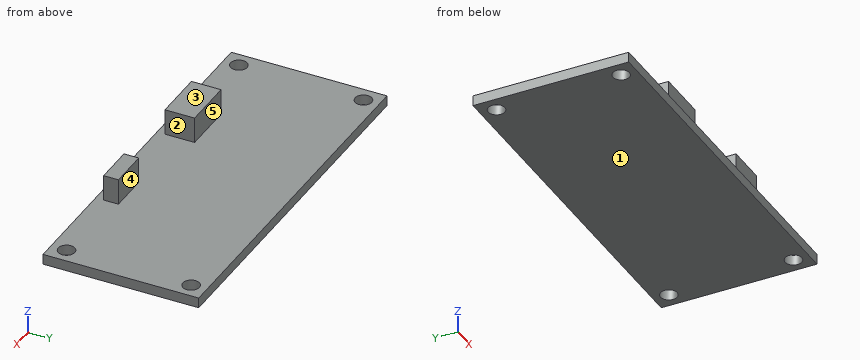
```python
from build123d import *

# Parameters (mm, degrees)
SKETCH_1_W      = 71
SKETCH_1_H      = 30
SKETCH_1_R      = 1.6
EXTRUDE_1_DEPTH = 2
SKETCH_2_W      = 9.975674075
SKETCH_2_H      = 5.707731043
SKETCH_2_W_2    = 7.661729058
SKETCH_2_H_2    = 2.853865522
EXTRUDE_2_DEPTH = 5


with BuildPart() as part:
    # 草图1 → 凸台-拉伸1 (new body)
    with BuildSketch(Plane.XY):
        with Locations((35.5, 15)):
            Rectangle(SKETCH_1_W, SKETCH_1_H)
        with Locations((3, 27)):
            Circle(SKETCH_1_R, mode=Mode.SUBTRACT)
        with Locations((68, 3)):
            Circle(SKETCH_1_R, mode=Mode.SUBTRACT)
        with Locations((3, 3)):
            Circle(SKETCH_1_R, mode=Mode.SUBTRACT)
        with Locations((68, 27)):
            Circle(SKETCH_1_R, mode=Mode.SUBTRACT)
    extrude(amount=EXTRUDE_1_DEPTH)

    # 草图2 → 凸台-拉伸2 (add)
    with BuildSketch(Plane.XY.offset(2)):
        with Locations((23.004696906, 4.381563419)):
            Rectangle(SKETCH_2_W, SKETCH_2_H)
        with Locations((47.301119589, 2.954630659)):
            Rectangle(SKETCH_2_W_2, SKETCH_2_H_2)
    extrude(amount=EXTRUDE_2_DEPTH)


solid = part.part
```
CAD build for the part. Positions are in the model's coordinates, mm. Face numbers are marked on the shaded views. A direction names the side the tool comes from. Coordinates: 2 decimals unless noted, no trailing zeros. Order: outer loops, then holes, each group sorted by start corner. A loop starts at its lowest first (then second) coordinate and runs counter-clockwise, first axis right, second up. Notation, with made-up numbers: M 27.25,-8 L 83.25,-8 A11 cw 83.25,0 Z; hole C 1,57 d9. An arc over 180 degrees is marked long. Write each question's results on one line, items separated by ' | '. Start each with the question number.
Q1. Cut at B-B (y = 27). List the corners of the cut face in (x, z), then the cut area to 3 significant figures.
Q2. Cut at C-C (z = 3). List the corners of the cut face in (x, y), then the cut area to 3 significant figures.
Q3. Cut at A-A (x = 68). List the corners of the cut face in (y, z).
Q4. Which spindle directions (+Z, -Z, +X, -X, +Y, -Y) get a long thin tool onto all of the face, cutting with end or side? Do the marked faces 3, 4 and 5. Say none if no direction does.
Q5. Drill centre lines: probe 1 along Y at (x, z) = (3, 1.3); probe 2 along Z at (x, y) = (52, 15.5); probe 3 along X at (y, z) = (3.25, 6.5). Where is each one in solid material? Low to high. Write a range as from..to.
Q6. Flat gauge pins, fed straight in: P1, Ø2, axis at x = 8.5, z = 3.5, coming from the -Y side; P2, Ø1, axis at x = 34, y = 26, coming from the +Z side; P3, Ø0.9, axis at y = 3.5, z = 3.5, coming from the +X side; P4, Ø1.5, axis at x = 48, z = 4.5, coming from the +Y side. Where does each tip first touch, or does it go through?
Q7. Cut at D-D (x = 48). List the corners of the cut face in (y, z).
Q8. Pull direction X, two halves, no side cores. Call the marked faces 1 and 2: +X half, -X half, draft (parallel to the pull), parting line (faces both ways), or undercut.
Found:
1) outline: M 0,0 L 1.4,0 L 1.4,2 L 0,2 Z; M 4.6,0 L 66.4,0 L 66.4,2 L 4.6,2 Z; M 69.6,0 L 71,0 L 71,2 L 69.6,2 Z | area: 129 mm²
2) outline: M 18.02,1.53 L 27.99,1.53 L 27.99,7.24 L 18.02,7.24 Z; M 43.47,1.53 L 51.13,1.53 L 51.13,4.38 L 43.47,4.38 Z | area: 78.8 mm²
3) outline: M 0,0 L 1.4,0 L 1.4,2 L 0,2 Z; M 4.6,0 L 25.4,0 L 25.4,2 L 4.6,2 Z; M 28.6,0 L 30,0 L 30,2 L 28.6,2 Z
4) face 3: +Z, +X, -X, +Y, -Y | face 4: +Z, +X, +Y | face 5: +Z, +X, -X, +Y
5) probe 1: 0..1.4, 4.6..25.4, 28.6..30 | probe 2: 0..2 | probe 3: 18.02..27.99, 43.47..51.13
6) P1: through | P2: z = 2 | P3: x = 51.13 | P4: y = 4.38
7) outline: M 0,0 L 30,0 L 30,2 L 4.38,2 L 4.38,7 L 1.53,7 L 1.53,2 L 0,2 Z
8) face 1: draft | face 2: undercut
